Model file for the job. Use its own axes, mm. A direction names the side the tool comes from. Round coordinates to 2 decimals unless told otherwise and drop trailing zeros. Loops run counter-clockwise (first coordinate to the right, second up) from the corner with the lowest first, then second, coordinate; pieces in that order, holes last. Notation, with made-up numbers: (-2, 16.5) - (28, 16.5) arc R9 ccw to (28, 29.5) - close; hole circle Ø11 at (-29.75, 43). An arc over 180 degrees is marked (long way). Answer as a JSON object with one key per item and string values.
from build123d import *

# Parameters (mm, degrees)
SKETCH1_R           = 5
BOSS_EXTRUDE1_DEPTH = 6


with BuildPart() as part:
    # Sketch1 → Boss-Extrude1 (new body)
    with BuildSketch(Plane(origin=(0, 0, 0), x_dir=(1, 0, 0), z_dir=(0, 1, 0))):
        with BuildLine():
            Line((17.615827491, 6.405693798), (17.615827491, 7.364453077))
            Line((17.615827491, 7.364453077), (-1.545270838, 7.364453077))
            Line((-1.545270838, 7.364453077), (-1.545270838, 19.364453077))
            Line((-1.545270838, 19.364453077), (4.454729162, 19.364453077))
            Line((4.454729162, 19.364453077), (4.454729162, 23.311113477))
            Line((4.454729162, 23.311113477), (37.351818757, 23.311113477))
            Line((37.351818757, 23.311113477), (37.351818757, 29.311113477))
            Line((37.351818757, 29.311113477), (56.351818757, 29.311113477))
            Line((56.351818757, 29.311113477), (56.351818757, 23.311113477))
            Line((56.351818757, 23.311113477), (89.248908352, 23.311113477))
            Line((89.248908352, 23.311113477), (89.248908352, 19.364453077))
            Line((89.248908352, 19.364453077), (95.248908352, 19.364453077))
            Line((95.248908352, 19.364453077), (95.248908352, 7.364453077))
            Line((95.248908352, 7.364453077), (76.087810024, 7.364453077))
            Line((76.087810024, 7.364453077), (76.087810024, 6.405693798))
            ThreePointArc((76.087810024, 6.405693798), (74.330450711, 2.163053111), (70.087810024, 0.405693798))
            Line((70.087810024, 0.405693798), (53.496778433, 0.405693798))
            Line((53.496778433, 0.405693798), (53.496778433, 20.432362651))
            Line((53.496778433, 20.432362651), (40.206859082, 20.432362651))
            Line((40.206859082, 20.432362651), (40.206859082, 0.405693798))
            Line((40.206859082, 0.405693798), (23.615827491, 0.405693798))
            ThreePointArc((23.615827491, 0.405693798), (19.373186804, 2.163053111), (17.615827491, 6.405693798))
        make_face()
        with Locations(Location((28.974519722, 7.237839647, 0), (0, 0, 270))):
            Circle(SKETCH1_R, mode=Mode.SUBTRACT)
        with Locations(Location((64.729117792, 7.237839647, 0), (0, 0, 270))):
            Circle(SKETCH1_R, mode=Mode.SUBTRACT)
    extrude(amount=BOSS_EXTRUDE1_DEPTH)


solid = part.part
1) Tool access for faces 4 (the flat face through (86, 3, -7.364)), 5 (the flat face through (73, 3, -23.311)), 6 (the flat face through (21, 3, -23.311)), 7 (the flat face through (8, 3, -7.364)): list every direction of +Z, -Z, +X, -X, +Y, -Y with a clear straight run to the whole face (end or side of a thin tool).
Values follow:
{"face 4": "+Z, +X, +Y, -Y", "face 5": "-Z, +X, +Y, -Y", "face 6": "-Z, -X, +Y, -Y", "face 7": "+Z, -X, +Y, -Y"}
2) Slice it at C-C on y = 4.3. List the corners of the cut face in (x, z), then the cut area to 3 significant figures.
Values follow:
{"outline": "(-1.55, -19.36) - (4.45, -19.36) - (4.45, -23.31) - (37.35, -23.31) - (37.35, -29.31) - (56.35, -29.31) - (56.35, -23.31) - (89.25, -23.31) - (89.25, -19.36) - (95.25, -19.36) - (95.25, -7.36) - (76.09, -7.36) - (76.09, -6.41) arc R6 ccw to (70.09, -0.41) - (53.5, -0.41) - (53.5, -20.43) - (40.21, -20.43) - (40.21, -0.41) - (23.62, -0.41) arc R6 ccw to (17.62, -6.41) - (17.62, -7.36) - (-1.55, -7.36) - close; hole circle Ø10 at (28.97, -7.24); hole circle Ø10 at (64.73, -7.24)", "area": "1,580 mm²"}
3) Slice it at D-D on z = -5.5. List the corners of the cut face in (x, y).
Values follow:
{"outline": "(17.68, 0) - (24.29, 0) - (24.29, 6) - (17.68, 6) - close; (33.66, 0) - (40.21, 0) - (40.21, 6) - (33.66, 6) - close; (53.5, 0) - (60.04, 0) - (60.04, 6) - (53.5, 6) - close; (69.42, 0) - (76.02, 0) - (76.02, 6) - (69.42, 6) - close"}
4) Drop flat-ended pins along their axis: P1, Ø2, axis at y = 2, z = -20.5, coming from the +X side; P2, Ø1.8, axis at x = 46, y = 4, coming from the +Z side; P3, Ø1.1, axis at y = 3, z = -7, coming from the +X side; P4, Ø1.8, axis at x = 28, y = 4, coming from the -Z side. Give the stop position or say it passes through.
Values follow:
{"P1": "x = 89.25", "P2": "z = -20.43", "P3": "x = 95.25", "P4": "z = -23.31"}
5) Probe probe 1 along X at (y, z) = (0.35, -7.5); probe 2 along X at (y, z) = (4.6, -7.25); probe 3 along Z at (x, y) = (3.5, 5.5). List the from-to ranges inside material, lowest first.
Values follow:
{"probe 1": "-1.55 to 23.98, 33.97 to 40.21, 53.5 to 59.74, 69.72 to 95.25", "probe 2": "17.62 to 23.97, 33.97 to 40.21, 53.5 to 59.73, 69.73 to 76.09", "probe 3": "-19.36 to -7.36"}
6) Two-plate mould, pull along X, no slides. Class faces 1 (the cylindrical face through (74.377, 2.958, -2.21)), 2 (the cylindrical face through (19.42, 2.958, -2.117)), 3 (the flat face through (47, 3, -20.432)): pulls with the +X half, pulls with the -X half, needs draft (parallel to the pull), parting line crosses it, or undercut.
Values follow:
{"face 1": "pulls with the +X half", "face 2": "pulls with the -X half", "face 3": "undercut"}
7) Slice it at B-B on x = 25. List the corners of the cut face in (y, z).
Values follow:
{"outline": "(0, -23.31) - (6, -23.31) - (6, -10.27) - (0, -10.27) - close; (0, -4.2) - (6, -4.2) - (6, -0.41) - (0, -0.41) - close"}
8) Slice it at A-A on z = -14.5. List the corners of the cut face in (x, y), then the cut area to 3 significant figures.
Values follow:
{"outline": "(-1.55, 0) - (40.21, 0) - (40.21, 6) - (-1.55, 6) - close; (53.5, 0) - (95.25, 0) - (95.25, 6) - (53.5, 6) - close", "area": "501 mm²"}
